Part model, mm, in its own coordinate system. A direction names the side the tool comes from. Round coordinates to 2 decimals unless told otherwise and drop trailing zeros. Write each loop counter-clockwise with the first axis right and the second up, starting at its lowest first coordinate (ties: lowest second). Pieces come first, ordered by that corner, then holes. Notation, with made-up numbers: M 72.5,22 L 98.5,22 A7 cw 98.5,28 Z; hole C 8,66.5 d1. An arc over 180 degrees is marked long. Use a Markdown table: item, result. Add a question column.
1) Wall check: probe 1 along Y at (x, z) = (145, 4.5); probe 2 along Z at (x, y) = (43.75, 61.5); probe 3 along Y at (x, z) = (30.75, 5). Give the ranges that are in metal, low to high.
2) Drop flat-ended pins along their axis: P1, Ø4, axis at y = 63, z = 6.5, coming from the -X side; P2, Ø4.5, axis at x = 175, y = 13, coming from the -Z side; P3, Ø7, axis at y = 59.5, z = 14.5, coming from the -X side; P4, Ø2.5, axis at y = 61.5, z = 5, coming from the -X side. Give the stop position or say it passes through.
3) Two-plate mould, pull along X, no slides. Class faces 1 (the face through (20, 61, 10)), 2 (the face through (37.1, 4.1, 15.09)), 3 (the face through (27, 66, 10)): released by +X, released by -X, zero draft, split by the parting line, or undercut.
4) Which spindle directions (+Z, -Z, +X, -X, +Y, -Y) get a long thin tool onto all of the face, cutting with end or side? Do faces 4 (the face through (4.97, 30.95, 14.54)), 5 (the face through (5, 52, 10)), 6 (the face through (35.7, 62, 10)). Say none if no direction does.
5) Slice it at A-A on y = 53. Write the cut outline in (x, z), plus the area to 3 significant figures.
6) Slice it at B-B on x = 53. Write the cut outline in (y, z), plus the area to 3 significant figures.
7) Slice it at C-C on y = 18. Write the cut outline in (x, z), plus the area to 3 significant figures.
8) Slice it at D-D on x = 160. Write the cut outline in (y, z).
```python
from build123d import *

# Parameters (mm, degrees)
SKETCH_1_W              = 190
SKETCH_1_H              = 66
EXTRUDE_1_DEPTH         = 20
SKETCH_2_R              = 25
CUT_EXTRUDE_1_DEPTH     = 203.12867189
SKETCH_3_W              = 20
SKETCH_3_H              = 9
CUT_EXTRUDE_2_DEPTH     = 203.12867189
SKETCH_4_W              = 1.4
SKETCH_4_H              = 16.93413418
CUT_EXTRUDE_3_DEPTH     = 203.12867189
CHAMFER_1_SIZE          = 10
SKETCH_5_R              = 2.25
CUT_EXTRUDE_4_DEPTH     = 14.3
HOLE_WIZARD_M4_1_D      = 3.3
HOLE_WIZARD_M4_1_DEPTH  = 10.1
HOLE_WIZARD_M4_1_TIP    = 0.991420021
HOLE_WIZARD_M5_1_REACH  = 204.129
HOLE_WIZARD_M5_1_BORE_R = 2.1
HOLE_WIZARD_M5_2_D      = 4.2
HOLE_WIZARD_M5_2_DEPTH  = 12.4
HOLE_WIZARD_M5_2_TIP    = 1.2618073
CHAMFER_2_SIZE          = 10
HOLE_WIZARD_M6_1_D      = 5
PATTERN_LINEAR_1_COUNT  = 3
PATTERN_LINEAR_1_PITCH  = 15


with BuildPart() as part:
    # 草图1 → 凸台-拉伸1 (new body)
    with BuildSketch(Plane.XY):
        with Locations((95, 33)):
            Rectangle(SKETCH_1_W, SKETCH_1_H)
    extrude(amount=EXTRUDE_1_DEPTH)

    # 草图2 → 切除-拉伸1 (cut, through all)
    with BuildSketch(Plane(origin=(0, 0, 0), x_dir=(-1, 0, 0), z_dir=(0, 0, -1))):
        with Locations((-35, 33)):
            Circle(SKETCH_2_R)
    extrude(amount=-CUT_EXTRUDE_1_DEPTH, mode=Mode.SUBTRACT)

    # 草图3 → 切除-拉伸2 (cut, through all)
    with BuildSketch(Plane(origin=(0, 0, 0), x_dir=(-1, 0, 0), z_dir=(0, 0, -1))):
        with Locations((-10, 61.5)):
            Rectangle(SKETCH_3_W, SKETCH_3_H)
    extrude(amount=-CUT_EXTRUDE_2_DEPTH, mode=Mode.SUBTRACT)

    # 草图4 → 切除-拉伸3 (cut, through all)
    with BuildSketch(Plane(origin=(0, 0, 0), x_dir=(-1, 0, 0), z_dir=(0, 0, -1))):
        with Locations((-35, 57.53293291)):
            Rectangle(SKETCH_4_W, SKETCH_4_H)
    extrude(amount=-CUT_EXTRUDE_3_DEPTH, mode=Mode.SUBTRACT)

    # 倒角1
    chamfer_1_edges = [part.edges().sort_by_distance(p)[0] for p in [
        (0, 57, 10),
    ]]
    chamfer(chamfer_1_edges, length=CHAMFER_1_SIZE)

    # 草图5 → 切除-拉伸4 (cut)
    with BuildSketch(Plane.ZY.offset(-20)):
        with Locations(Location((15, 61.5, 0), (0, 0, 270))):
            Circle(SKETCH_5_R)
        with Locations((5, 61.5)):
            Circle(SKETCH_5_R)
    extrude(amount=-CUT_EXTRUDE_4_DEPTH, mode=Mode.SUBTRACT)

    # M4 螺纹孔1
    with Locations(Plane.ZY.offset(-35.7)):
        with Locations((15, 61.5), (5, 61.5)):
            Hole(HOLE_WIZARD_M4_1_D / 2, depth=HOLE_WIZARD_M4_1_DEPTH)
            with Locations((0, 0, -(HOLE_WIZARD_M4_1_DEPTH + HOLE_WIZARD_M4_1_TIP / 2))):  # 118° drill point
                Cone(0, HOLE_WIZARD_M4_1_D / 2, HOLE_WIZARD_M4_1_TIP, mode=Mode.SUBTRACT)

    # M5 螺纹孔1 bore → M5 螺纹孔1 (cut, up to next)
    with BuildSketch(Plane.ZY, mode=Mode.PRIVATE) as hole_wizard_m5_1_sk1:
        with Locations((15, 33)):
            Circle(HOLE_WIZARD_M5_1_BORE_R)
    hole_wizard_m5_1_tool1 = extrude(hole_wizard_m5_1_sk1.sketch, amount=-HOLE_WIZARD_M5_1_REACH, mode=Mode.PRIVATE) & part.part
    add(hole_wizard_m5_1_tool1.solids().sort_by_distance((0, 33, 15))[0], mode=Mode.SUBTRACT)

    # M5 螺纹孔2
    with Locations(Plane.XZ):
        with Locations((35, 15)):
            Hole(HOLE_WIZARD_M5_2_D / 2, depth=HOLE_WIZARD_M5_2_DEPTH)
            with Locations((0, 0, -(HOLE_WIZARD_M5_2_DEPTH + HOLE_WIZARD_M5_2_TIP / 2))):  # 118° drill point
                Cone(0, HOLE_WIZARD_M5_2_D / 2, HOLE_WIZARD_M5_2_TIP, mode=Mode.SUBTRACT)

    # 倒角2
    chamfer_2_edges = [part.edges().sort_by_distance(p)[0] for p in [
        (0, 0, 10),
    ]]
    chamfer(chamfer_2_edges, length=CHAMFER_2_SIZE)

    # M6 螺纹孔1 (through all)
    with Locations(Plane(origin=(0, 0, 0), x_dir=(-1, 0, 0), z_dir=(0, 0, -1))):
        with Locations((-175, 53), (-175, 13)):
            hole_wizard_m6_1 = Hole(HOLE_WIZARD_M6_1_D / 2)

    # 阵列(线性)1: M6 螺纹孔1 ×3
    with Locations(*[(-i * PATTERN_LINEAR_1_PITCH, 0, 0) for i in range(1, PATTERN_LINEAR_1_COUNT)]):
        add(hole_wizard_m6_1, mode=Mode.SUBTRACT)


solid = part.part
```
Entries:
| question | item | result |
|---|---|---|
| 1 | probe 1 | y = 0 to 10.5, 15.5 to 50.5, 55.5 to 66 |
| 1 | probe 2 | z = 0 to 3.35, 6.65 to 13.35, 16.65 to 20 |
| 1 | probe 3 | y = 0 to 8.36, 57.64 to 59.25, 63.75 to 66 |
| 2 | P1 | stops at x = 20 |
| 2 | P2 | passes through |
| 2 | P3 | stops at x = 9 |
| 2 | P4 | stops at x = 46.04 |
| 3 | face 1 | released by -X |
| 3 | face 2 | undercut |
| 3 | face 3 | zero draft |
| 4 | face 4 | -X |
| 4 | face 5 | +Z, -Z, -X, +Y |
| 4 | face 6 | +Z, -Z, +Y |
| 5 | outline | M 6,0 L 20,0 L 20,20 L 6,20 Z; M 50,0 L 142.5,0 L 142.5,20 L 50,20 Z; M 147.5,0 L 157.5,0 L 157.5,20 L 147.5,20 Z; M 162.5,0 L 172.5,0 L 172.5,20 L 162.5,20 Z; M 177.5,0 L 190,0 L 190,20 L 177.5,20 Z |
| 5 | area | 2,780 mm^2 |
| 6 | outline | M 0,0 L 15.65,0 L 15.65,20 L 0,20 Z; M 50.35,0 L 66,0 L 66,20 L 50.35,20 Z |
| 6 | area | 626 mm^2 |
| 7 | outline | M 0,0 L 15,0 L 15,20 L 0,20 Z; M 55,0 L 190,0 L 190,20 L 55,20 Z |
| 7 | area | 3,000 mm^2 |
| 8 | outline | M 0,0 L 10.5,0 L 10.5,20 L 0,20 Z; M 15.5,0 L 50.5,0 L 50.5,20 L 15.5,20 Z; M 55.5,0 L 66,0 L 66,20 L 55.5,20 Z |
